```python
from build123d import *

# Parameters (mm, degrees)
SKETCH1_W           = 152.4
SKETCH1_H           = 101.6
BOSS_EXTRUDE1_DEPTH = 31.75
CUT_EXTRUDE1_DEPTH  = 28.575
SKETCH3_W           = 4.7625
SKETCH3_H           = 6.35
CUT_EXTRUDE2_DEPTH  = 26.9875


with BuildPart() as part:
    # Sketch1 → Boss-Extrude1 (new body)
    with BuildSketch(Plane(origin=(0, 0, 0), x_dir=(1, 0, 0), z_dir=(0, 1, 0))):
        Rectangle(SKETCH1_W, SKETCH1_H)
    extrude(amount=BOSS_EXTRUDE1_DEPTH)

    # Sketch2 → Cut-Extrude1 (cut)
    with BuildSketch(Plane(origin=(0, 31.75, 0), x_dir=(1, 0, 0), z_dir=(0, 1, 0))):
        Polygon((71.4375, -46.0375), (-71.4375, -46.0375), (-71.4375, 46.0375), (71.4375, 46.0375), (80.9625, 46.0375), (80.9625, -46.0375), align=None)
    extrude(amount=-CUT_EXTRUDE1_DEPTH, mode=Mode.SUBTRACT)

    # Sketch3 → Cut-Extrude2 (cut)
    with BuildSketch(Plane(origin=(76.2, 0, 0), x_dir=(0, 0, -1), z_dir=(1, 0, 0))):
        with Locations((-46.83125, 25.4)):
            Rectangle(SKETCH3_W, SKETCH3_H)
        with Locations((46.83125, 25.4)):
            Rectangle(SKETCH3_W, SKETCH3_H)
    extrude(amount=-CUT_EXTRUDE2_DEPTH, mode=Mode.SUBTRACT)


solid = part.part
```
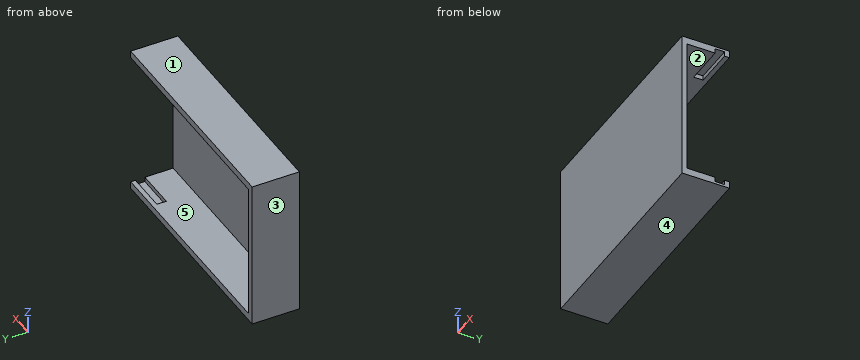
The listing builds one solid part. Answer for the finished solid, in the listing's coordinates (mm). Face numbers are marked on the shaded views. A direction names the side the tool comes from. Round coordinates to 2 decimals unless told otherwise and drop trailing zeros. Write each loop counter-clockwise with the first axis right and the second up, starting at its lowest first coordinate (ties: lowest second). Pieces come first, ordered by that corner, then holes. Notation, with made-up numbers: (35.25, 83) -> (78.25, 83) arc R28 cw to (78.25, 115) -> close; hole circle Ø11 at (-28.75, -39.75). An arc over 180 degrees is marked (long way). Answer as a JSON object with one key per item and string values. Group by question number.
Q1. Section B-B (y = 26.5) is taken. Write down the section's boundary in (x, z).
Q2. Each of these flat-tipped pins is pushed along its axis until it touches: pin 1 Ø2 at (x, z) = (25.5, 14) entering from -Y; pin 2 Ø10 at (x, z) = (12.5, 9.5) entering from +Y (3 decimals). Where does it stop, or does it pass through?
Q3. Which of the six approach directions +Z, -Z, +X, -X, +Y, -Y give full straight-line access (tool end or side, diameter ignored) to the marked faces 4 and 5?
Q4. Determine the mould class of the marked faces 1, 2 and 3 for opening direction Z: pulls with the +Z half, pulls with the -Z half, needs draft (parallel to the pull), parting line crosses it, or undercut.
Q5. Straight lines are drawn through the part: line 1 along Z through (x, y) = (4.5, 14); line 2 along Z through (x, y) = (69, 23.5); line 3 along X through (y, z) = (10, -13). For each, find the intervals that lie inside material, in ascending order.
Check values:
{
 "1": {"outline": "(-76.2, -50.8) -> (76.2, -50.8) -> (76.2, -49.21) -> (49.21, -49.21) -> (49.21, -46.04) -> (-71.44, -46.04) -> (-71.44, 46.04) -> (49.21, 46.04) -> (49.21, 49.21) -> (76.2, 49.21) -> (76.2, 50.8) -> (-76.2, 50.8) -> close"},
 "2": {"pin 1": "y = 0", "pin 2": "y = 3.175"},
 "3": {"face 4": "-Z, +X, -X, +Y, -Y", "face 5": "+X, +Y"},
 "4": {"face 1": "pulls with the +Z half", "face 2": "undercut", "face 3": "needs draft"},
 "5": {"line 1": "-50.8 to -46.04, 46.04 to 50.8", "line 2": "-50.8 to -49.21, 49.21 to 50.8", "line 3": "-76.2 to -71.44"}
}
